Can you work these out from the model? Positions are in its coordinate system, mm. Coordinates: 2 decimals unless noted, no trailing zeros. Write each loop counter-clockwise with the first axis right and the second up, starting at its lowest first coordinate (ties: lowest second). Pieces come first, ordered by that corner, then holes. Notation, with made-up numbers: (30, -34.5) - (52, -34.5) arc R21 ccw to (52, -17.5) - close; hole circle Ø3 at (-22.75, 43). An arc over 180 degrees is marked (long way). Use one line per item in the form item = value. Start each with the question number.
(1) If I drill on probe 1 along Z at (x, y) = (75, 4.75), over which ranges is the centre line in solid material (lowest first)? Write a range as from..to.
(2) For pin 1 Ø1.5 at (x, y) = (201, 5) entering from +Z; pin 2 Ø1.9 at (y, z) = (2, 73) entering from +X; pin 3 Ø1.9 at (y, z) = (2, 72) entering from -X, each with a flat end and sliding along its axis, tell me the tip position at first contact or that it passes through.
(3) If we section it at A-A on x = -220.5: Please give me the cut outline in (y, z), then the cut area to 3 significant figures.
```python
from build123d import *

# Parameters (mm, degrees)
SKETCH1_W                 = 721.63658441
SKETCH1_H                 = 152.4
BOSS_EXTRUDE1_DEPTH       = 6.35
SKETCH2_W                 = 39.679316882
SKETCH2_H                 = 6.35
SKETCH2_W_2               = 31.750000127
CUT_EXTRUDE1_DEPTH        = 7.35
LPATTERN1_COUNT           = 3
LPATTERN1_PITCH           = 153.979316882
LPATTERN1_COL_COUNT       = 3
LPATTERN1_COL_PITCH       = 153.979316882
MIRROR1_COPY_1_SKETCH_W   = 39.679316882
MIRROR1_COPY_1_SKETCH_H   = 6.35
MIRROR1_COPY_1_SKETCH_W_2 = 31.750000127
MIRROR1_COPY_1_DEPTH      = 7.35
MIRROR1_COPY_2_SKETCH_W   = 39.679316882
MIRROR1_COPY_2_SKETCH_H   = 6.35
MIRROR1_COPY_2_SKETCH_W_2 = 31.750000127
MIRROR1_COPY_2_DEPTH      = 7.35
MIRROR1_COPY_3_SKETCH_W   = 39.679316882
MIRROR1_COPY_3_SKETCH_H   = 6.35
MIRROR1_COPY_3_SKETCH_W_2 = 31.750000127
MIRROR1_COPY_3_DEPTH      = 7.35
MIRROR1_COPY_4_SKETCH_W   = 39.679316882
MIRROR1_COPY_4_SKETCH_H   = 6.35
MIRROR1_COPY_4_SKETCH_W_2 = 31.750000127
MIRROR1_COPY_4_DEPTH      = 7.35


with BuildPart() as part:
    # Sketch1 → Boss-Extrude1 (new body)
    with BuildSketch(Plane(origin=(0, 0, 0), x_dir=(1, 0, 0), z_dir=(0, 1, 0))):
        Rectangle(SKETCH1_W, SKETCH1_H)
    extrude(amount=BOSS_EXTRUDE1_DEPTH)

    # Sketch2 → Cut-Extrude1 (cut, through all)
    with BuildSketch(Plane(origin=(0, 6.35, 0), x_dir=(1, 0, 0), z_dir=(0, 1, 0))):
        with Locations((0, -73.025)):
            Rectangle(SKETCH2_W, SKETCH2_H)
        with Locations((-61.114658505, -73.025)):
            Rectangle(SKETCH2_W_2, SKETCH2_H)
        with Locations((61.114658505, -73.025)):
            Rectangle(SKETCH2_W_2, SKETCH2_H)
    cut_extrude1 = extrude(amount=-CUT_EXTRUDE1_DEPTH, mode=Mode.SUBTRACT)

    # LPattern1: Cut-Extrude1 ×3
    with Locations(*[(i * LPATTERN1_PITCH, 0, 0) for i in range(1, LPATTERN1_COUNT)]):
        add(cut_extrude1, mode=Mode.SUBTRACT)

    # LPattern1 col: Cut-Extrude1 ×3
    with Locations(*[(-i * LPATTERN1_COL_PITCH, 0, 0) for i in range(1, LPATTERN1_COL_COUNT)]):
        add(cut_extrude1, mode=Mode.SUBTRACT)

    # Mirror1: Cut-Extrude1 across plane
    add(cut_extrude1.mirror(Plane.XY), mode=Mode.SUBTRACT)

    # Mirror1 copy 1 sketch → Mirror1 copy 1 (cut, through all)
    with BuildSketch(Plane(origin=(153.979316882, 6.35, 0), x_dir=(1, 0, 0), z_dir=(0, 1, 0))):
        with Locations((0, 73.025)):
            Rectangle(MIRROR1_COPY_1_SKETCH_W, MIRROR1_COPY_1_SKETCH_H)
        with Locations((-61.114658505, 73.025)):
            Rectangle(MIRROR1_COPY_1_SKETCH_W_2, MIRROR1_COPY_1_SKETCH_H)
        with Locations((61.114658505, 73.025)):
            Rectangle(MIRROR1_COPY_1_SKETCH_W_2, MIRROR1_COPY_1_SKETCH_H)
    extrude(amount=-MIRROR1_COPY_1_DEPTH, mode=Mode.SUBTRACT)

    # Mirror1 copy 2 sketch → Mirror1 copy 2 (cut, through all)
    with BuildSketch(Plane(origin=(307.958633764, 6.35, 0), x_dir=(1, 0, 0), z_dir=(0, 1, 0))):
        with Locations((0, 73.025)):
            Rectangle(MIRROR1_COPY_2_SKETCH_W, MIRROR1_COPY_2_SKETCH_H)
        with Locations((-61.114658505, 73.025)):
            Rectangle(MIRROR1_COPY_2_SKETCH_W_2, MIRROR1_COPY_2_SKETCH_H)
        with Locations((61.114658505, 73.025)):
            Rectangle(MIRROR1_COPY_2_SKETCH_W_2, MIRROR1_COPY_2_SKETCH_H)
    extrude(amount=-MIRROR1_COPY_2_DEPTH, mode=Mode.SUBTRACT)

    # Mirror1 copy 3 sketch → Mirror1 copy 3 (cut, through all)
    with BuildSketch(Plane(origin=(-153.979316882, 6.35, 0), x_dir=(1, 0, 0), z_dir=(0, 1, 0))):
        with Locations((0, 73.025)):
            Rectangle(MIRROR1_COPY_3_SKETCH_W, MIRROR1_COPY_3_SKETCH_H)
        with Locations((-61.114658505, 73.025)):
            Rectangle(MIRROR1_COPY_3_SKETCH_W_2, MIRROR1_COPY_3_SKETCH_H)
        with Locations((61.114658505, 73.025)):
            Rectangle(MIRROR1_COPY_3_SKETCH_W_2, MIRROR1_COPY_3_SKETCH_H)
    extrude(amount=-MIRROR1_COPY_3_DEPTH, mode=Mode.SUBTRACT)

    # Mirror1 copy 4 sketch → Mirror1 copy 4 (cut, through all)
    with BuildSketch(Plane(origin=(-307.958633764, 6.35, 0), x_dir=(1, 0, 0), z_dir=(0, 1, 0))):
        with Locations((0, 73.025)):
            Rectangle(MIRROR1_COPY_4_SKETCH_W, MIRROR1_COPY_4_SKETCH_H)
        with Locations((-61.114658505, 73.025)):
            Rectangle(MIRROR1_COPY_4_SKETCH_W_2, MIRROR1_COPY_4_SKETCH_H)
        with Locations((61.114658505, 73.025)):
            Rectangle(MIRROR1_COPY_4_SKETCH_W_2, MIRROR1_COPY_4_SKETCH_H)
    extrude(amount=-MIRROR1_COPY_4_DEPTH, mode=Mode.SUBTRACT)


solid = part.part
```
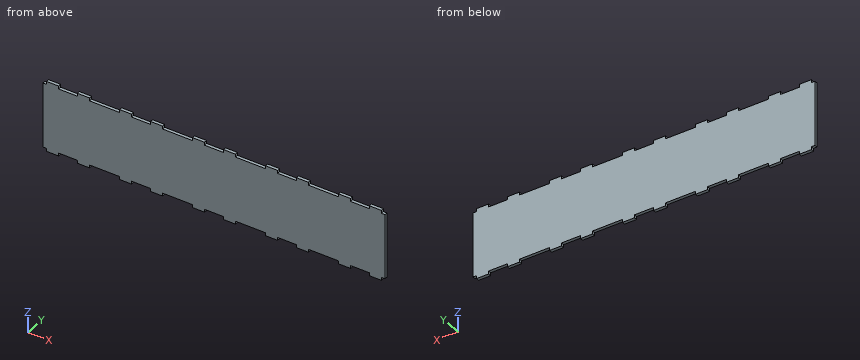
Reported:
q1.probe_1 = -69.85..69.85
q2.pin_1 = 69.85
q2.pin_2 = 353.2
q2.pin_3 = -353.2
q3.outline = (0, -69.85) - (6.35, -69.85) - (6.35, 69.85) - (0, 69.85) - close
q3.area = 887 mm2
